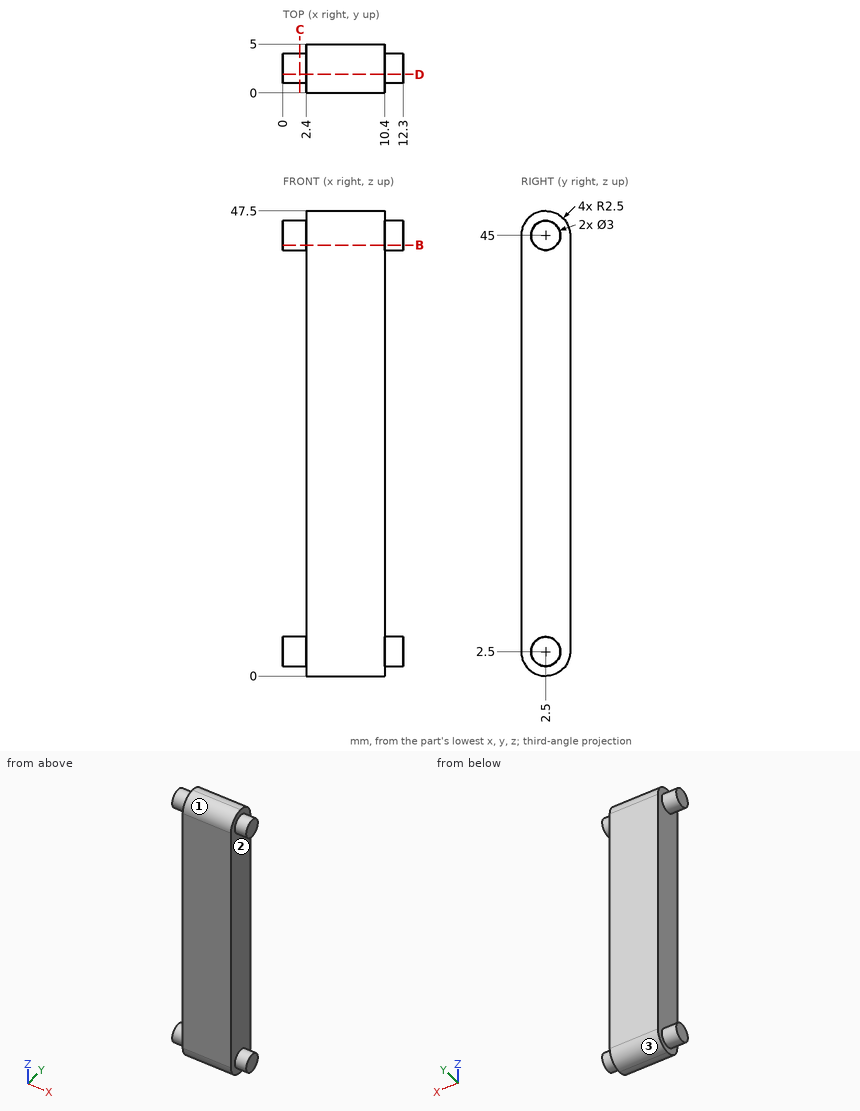
Input: dimensioned drawing with shaded views. Units: mm. Origin: part minimum x, y, z. Round coordinates to 2 decimals unless told otherwise and drop trailing zeros. Loops run counter-clockwise (first coordinate to the right, second up) from the corner with the lowest first, then second, coordinate; pieces in that order, holes last. Notation, with made-up numbers: M 71,46.25 L 113,46.25 A17 ccw 113,52.25 Z; hole C 68.5,-15.75 d9. An arc over 180 degrees is marked long. Answer in a Markdown table with one row per item. Add a question column.
1. Mould query, pull axis Z, two halves, no side actions, for the marked faces 1, 2 and 3. Classes: released by +Z, released by -Z, zero draft, split by the parting line, or undercut.
2. Section D-D (y = 1.9). Output: boundary loops of the cut face in (x, z), and give its area (4 significant figures).
3. Section B-B (z = 44). Output: boundary loops of the cut face in (x, y), and give its area (3 significant figures).
4. Section C-C (x = 1.75). Output: boundary loops of the cut face in (y, z).
5. Ray query, probe 1 along X at (y, z) = (3.85, 37); probe 2 along Z at (x, y) = (2.25, 2.05); probe 3 along Z at (x, y) = (11.5, 3.3). Return the intervals inside material, ascending.
6. Contact query for flat-ended pins moving along their axis: pin 1 (3 mm diameter, centred on y = 1.5, z = 28.5, fed in from +X); pin 2 (1.5 mm diameter, centred on y = 1.5, z = 29, fed in from -X). Output: stop coordinate, or through.
Values follow:
| question | item | result |
|---|---|---|
| 1 | face 1 | released by +Z |
| 1 | face 2 | undercut |
| 1 | face 3 | released by -Z |
| 2 | outline | M 0,1.13 L 2.4,1.13 L 2.4,0.07 L 10.4,0.07 L 10.4,1.13 L 12.3,1.13 L 12.3,3.87 L 10.4,3.87 L 10.4,43.63 L 12.3,43.63 L 12.3,46.37 L 10.4,46.37 L 10.4,47.43 L 2.4,47.43 L 2.4,46.37 L 0,46.37 L 0,43.63 L 2.4,43.63 L 2.4,3.87 L 0,3.87 Z |
| 2 | area | 402.5 mm^2 |
| 3 | outline | M 0,1.38 L 2.4,1.38 L 2.4,0 L 10.4,0 L 10.4,1.38 L 12.3,1.38 L 12.3,3.62 L 10.4,3.62 L 10.4,5 L 2.4,5 L 2.4,3.62 L 0,3.62 Z |
| 3 | area | 49.6 mm^2 |
| 4 | outline | C 2.5,2.5 d3; C 2.5,45 d3 |
| 5 | probe 1 | 2.4 to 10.4 |
| 5 | probe 2 | 1.07 to 3.93, 43.57 to 46.43 |
| 5 | probe 3 | 1.23 to 3.77, 43.73 to 46.27 |
| 6 | pin 1 | x = 10.4 |
| 6 | pin 2 | x = 2.4 |
